Model file for the job. Use its own axes, mm. Face numbers are marked on the shaded views. A direction names the side the tool comes from. Give positions to 0.01 mm unless a question says otherwise; leave off trailing zeros. Write each loop counter-clockwise with the first axis right and the second up, starting at its lowest first coordinate (ties: lowest second). Pieces come first, ordered by that corner, then holes.
```python
from build123d import *

# Parameters (mm, degrees)
SKETCH3_R           = 70
BOSS_EXTRUDE1_DEPTH = 200
SKETCH4_R           = 19.75
BOSS_EXTRUDE2_DEPTH = 15
SKETCH5_R           = 31.5
BOSS_EXTRUDE3_DEPTH = 7
SKETCH6_R           = 13.005945397
SKETCH6_R_2         = 5.913103463
BOSS_EXTRUDE4_DEPTH = 10


with BuildPart() as part:
    # Sketch3 → Boss-Extrude1 (new body)
    with BuildSketch(Plane.XY):
        Circle(SKETCH3_R)
    extrude(amount=BOSS_EXTRUDE1_DEPTH)

    # Sketch4 → Boss-Extrude2 (add)
    with BuildSketch(Plane.XY.offset(200)):
        Circle(SKETCH4_R)
    extrude(amount=BOSS_EXTRUDE2_DEPTH)

    # Sketch5 → Boss-Extrude3 (add)
    with BuildSketch(Plane(origin=(0, 0, 0), x_dir=(-1, 0, 0), z_dir=(0, 0, -1))):
        with Locations(Location((0, 0, 0), (0, 0, 180))):
            Circle(SKETCH5_R)
    extrude(amount=BOSS_EXTRUDE3_DEPTH)

    # Sketch6 → Boss-Extrude4 (add)
    with BuildSketch(Plane(origin=(0, 0, -7), x_dir=(-1, 0, 0), z_dir=(0, 0, -1))):
        with Locations((8.337101301, 8.580168456)):
            Circle(SKETCH6_R)
        with Locations((-13.657956127, -10.615712672)):
            Circle(SKETCH6_R_2)
    extrude(amount=BOSS_EXTRUDE4_DEPTH)


solid = part.part
```
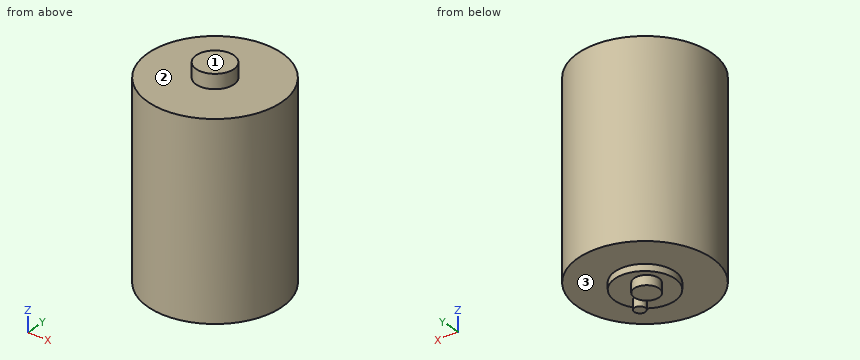
1. Slice it at C-C, the plane y = 0. Write the cut outline in (x, z).
Calculated:
outline: (-70, 0) - (-31.5, 0) - (-31.5, -7) - (-18.11, -7) - (-18.11, -17) - (1.44, -17) - (1.44, -7) - (31.5, -7) - (31.5, 0) - (70, 0) - (70, 200) - (19.75, 200) - (19.75, 215) - (-19.75, 215) - (-19.75, 200) - (-70, 200) - close
2. Which spindle directions (+Z, -Z, +X, -X, +Y, -Y) get a long thin tool onto all of the face, cutting with end or side? Do the marked faces 1, 2 and 3. Say none if no direction does.
Calculated:
face 1: +Z, +X, -X, +Y, -Y
face 2: +Z
face 3: -Z
3. Slice it at A-A, the plane x = 12. Write the cut outline in (y, z), and give its area (3 significant figures).
Calculated:
outline: (-68.96, 0) - (-29.12, 0) - (-29.12, -7) - (-16.29, -7) - (-16.29, -17) - (-4.94, -17) - (-4.94, -7) - (29.12, -7) - (29.12, 0) - (68.96, 0) - (68.96, 200) - (15.69, 200) - (15.69, 215) - (-15.69, 215) - (-15.69, 200) - (-68.96, 200) - close
area: 28,600 mm2
4. Slice it at D-D, the plane x = -24.5. Write the cut outline in (y, z), and give its area (3 significant figures).
Calculated:
outline: (-65.57, 0) - (-19.8, 0) - (-19.8, -7) - (19.8, -7) - (19.8, 0) - (65.57, 0) - (65.57, 200) - (-65.57, 200) - close
area: 26,500 mm2
5. Pin check, flat tips, straight feed: P1, Ø3, axis at x = -43, y = -9, coming from the -Z side; P2, Ø10, axis at x = 32.5, z = 83.5, coming from the -Y side; P3, Ø5, axis at x = -42, z = 165.5, coming from the +Y side. Stop position of each tip, or through.
Calculated:
P1: stops at z = 0
P2: stops at y = -64.37
P3: stops at y = 57.79
6. Slice it at B-B, the plane z = 66. Write the cut outline in (x, y), and give its area (3 significant figures).
Calculated:
outline: circle Ø140 at (0, 0)
area: 15,400 mm2
7. Probe probe 1 along Z at (x, y) = (34, -39.5); probe 2 along Y at (x, z) = (60.5, 60); probe 3 along Y at (x, z) = (-61, 10). List the from-to ranges inside material, lowest first.
Calculated:
probe 1: z = 0 to 200
probe 2: y = -35.21 to 35.21
probe 3: y = -34.34 to 34.34
